from build123d import *

# Parameters (mm, degrees)
SKETCH_1_R          = 6.1
EXTRUDE_1_DEPTH     = 20
SKETCH_2_R          = 1.6
CUT_EXTRUDE_1_DEPTH = 65.52906322
FILLET_1_R          = 2


with BuildPart() as part:
    # 草图1 → 凸台-拉伸1 (new body)
    with BuildSketch(Plane.XY):
        with BuildLine():
            Line((0, 0), (20, 0))
            Line((20, 0), (20, 30))
            Line((20, 30), (20, 48))
            ThreePointArc((20, 48), (10, 58), (0, 48))
            Line((0, 48), (0, 30))
            Line((0, 30), (0, 0))
        make_face()
        with Locations((10, 48)):
            Circle(SKETCH_1_R, mode=Mode.SUBTRACT)
    extrude(amount=EXTRUDE_1_DEPTH)

    # 草图2 → 切除-拉伸1 (cut, through all)
    with BuildSketch(Plane(origin=(20, 0, 0), x_dir=(0, 0, -1), z_dir=(1, 0, 0))):
        with Locations((-15, 24)):
            Circle(SKETCH_2_R)
        with Locations(Location((-15, 6, 0), (0, 0, 180))):
            Circle(SKETCH_2_R)
        with Locations((-5, 6)):
            Circle(SKETCH_2_R)
        with Locations(Location((-5, 24, 0), (0, 0, 180))):
            Circle(SKETCH_2_R)
    extrude(amount=-CUT_EXTRUDE_1_DEPTH, mode=Mode.SUBTRACT)

    # 圆角1
    fillet_1_edges = [part.edges().sort_by_distance(p)[0] for p in [
        (20, 0, 10),
        (0, 0, 10),
    ]]
    fillet(fillet_1_edges, radius=FILLET_1_R)


solid = part.part
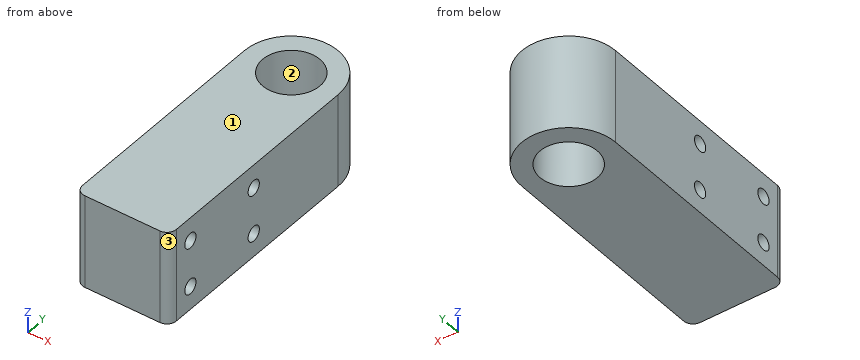
Source: CAD feature listing. Evaluate the final solid. Frame: model axes, mm. Face numbers are marked on the shaded views. Give positions to 0.01 mm unless a question says otherwise; leave off trailing zeros. Order: outer loops, then holes, each group sorted by start corner. A loop starts at its lowest first (then second) coordinate and runs counter-clockwise, first axis right, second up. Notation, with made-up numbers: (-11.5, 85.25) -> (20.5, 85.25) arc R29 ccw to (20.5, 113.25) -> close; hole circle Ø11 at (-17, 72). An arc over 180 degrees is marked (long way). Write item = value, one per line.
Q1. Pin query (flat end, axial travel): pin 1 (3 mm diameter, centred on x = 15, z = 12.5, fed in from +Y); pin 2 (4 mm diameter, centred on x = 7.5, z = 12.5, fed in from +Y). Return the tip coordinate at first contact, or that it passes through.
Data:
pin_1 = 57.37
pin_2 = 57.99
Q2. Material intervals for line 1 (Y direction, x = 9.25, z = 5); line 2 (Y direction, x = 11.5, z = 2); line 3 (Y direction, x = 4.75, z = 4), sorted ascending. Write a range as from..to.
Data:
line_1 = 0..4.4, 7.6..22.4, 25.6..41.95, 54.05..57.97
line_2 = 0..42.09, 53.91..57.89
line_3 = 0..4.75, 7.25..22.75, 25.25..44.89, 51.11..56.51
Q3. Cut plane D-D, the plane z = 9.75. Output: boundary loops of the cut face in (x, y).
Data:
outline = (0, 2) arc R2 ccw to (2, 0) -> (18, 0) arc R2 ccw to (20, 2) -> (20, 48) arc R10 ccw to (0, 48) -> close; hole circle Ø12.2 at (10, 48)
Q4. Pull-direction query (X, two-part tool) for the marked faces 1, 2 and 3; classes: released by +X, released by -X, zero draft, split by the parting line, or undercut.
Data:
face_1 = zero draft
face_2 = undercut
face_3 = released by +X
Q5. Cut plane A-A, the plane z = 15. Output: boundary loops of the cut face in (x, y).
Data:
outline = (0, 2) arc R2 ccw to (2, 0) -> (18, 0) arc R2 ccw to (20, 2) -> (20, 4.4) -> (0, 4.4) -> close; (0, 7.6) -> (20, 7.6) -> (20, 22.4) -> (0, 22.4) -> close; (0, 25.6) -> (20, 25.6) -> (20, 48) arc R10 ccw to (0, 48) -> close; hole circle Ø12.2 at (10, 48)
Q6. Cut plane B-B, the plane y = 24. Output: boundary loops of the cut face in (x, z).
Data:
outline = (0, 0) -> (20, 0) -> (20, 3.4) -> (0, 3.4) -> close; (0, 6.6) -> (20, 6.6) -> (20, 13.4) -> (0, 13.4) -> close; (0, 16.6) -> (20, 16.6) -> (20, 20) -> (0, 20) -> close
Q7. Cut plane C-C, the plane x = 10. Output: boundary loops of the cut face in (y, z), and give its area (3 significant figures).
Data:
outline = (0, 0) -> (41.9, 0) -> (41.9, 20) -> (0, 20) -> close; (54.1, 0) -> (58, 0) -> (58, 20) -> (54.1, 20) -> close; hole circle Ø3.2 at (6, 5); hole circle Ø3.2 at (6, 15); hole circle Ø3.2 at (24, 5); hole circle Ø3.2 at (24, 15)
area = 884 mm^2
